Work out the finished part from the listing and answer in its coordinate system (mm). A direction names the side the tool comes from. Round coordinates to 2 decimals unless told otherwise and drop trailing zeros. Write each loop counter-clockwise with the first axis right and the second up, starting at its lowest first coordinate (ties: lowest second). Pieces come first, ordered by that corner, then holes. Notation, with made-up numbers: M -15.5,-25 L 1.5,-25 A27 ccw 1.5,-7 Z; hole C -20.75,-26 d5. An arc over 180 degrees is marked long. One line per item, written item: value. Start each with the question number.
Q1. Find section A-A (x = 99.5). Write down the section's boundary in (y, z), and give its area (3 significant figures).
Q2. A tool of negligible diameter and unlimited length cuts with its end or side. For faces 4 (the flat face through (-5.5, 6, -65)), 5 (the flat face through (16, 6, 45.156)), 6 (the flat face through (57, 6, 45.156)), from which of +Z, -Z, +X, -X, +Y, -Y can it reach the whole face along a straight path? Write none if from no direction.
Q3. Consider probe 1 along X at (y, z) = (1.75, -117); probe 2 along X at (y, z) = (6, -40); probe 3 along Y at (x, z) = (11, 39). Determine where each line is inside the solid, lowest interval first.
Q4. Find section B-B (z = -69). Write down the section's boundary in (x, y), and give its area (3 significant figures).
Q5. Given pin 1 Ø3 at (x, y) = (12.5, 7) entering from +Z; pin 2 Ø1.8 at (y, z) = (6, 28.41) entering from +X; pin 3 Ø1.5 at (y, z) = (1.5, -28) entering from -X, each flat-ended and moving along its own axis, determine where each tip first touches the part or whether it passes through.
Q6. The mould has two halves that part along X. Classify faces 1 (the flat face through (73.5, 6, 40)), 2 (the flat face through (28, 6, 52)), 3 (the flat face through (-12, 6, -0.344)): released by +X, released by -X, zero draft, split by the parting line, or undercut.
from build123d import *

# Parameters (mm, degrees)
BOSS_EXTRUDE1_DEPTH = 12
SKETCH2_R           = 0.9921875
CUT_EXTRUDE1_DEPTH  = 12
SKETCH3_R           = 0.9921875
CUT_EXTRUDE2_DEPTH  = 12
SKETCH4_R           = 1
CUT_EXTRUDE3_DEPTH  = 219.054378342


with BuildPart() as part:
    # Sketch1 → Boss-Extrude1 (new body)
    with BuildSketch(Plane(origin=(0, 0, 0), x_dir=(1, 0, 0), z_dir=(0, 1, 0))):
        with BuildLine():
            Line((-5.5, 132.84375), (-5.5, 94.34375))
            Line((-5.5, 94.34375), (-17.5, 94.34375))
            Line((-17.5, 94.34375), (-17.5, 82.34375))
            Line((-17.5, 82.34375), (-5.5, 82.34375))
            Line((-5.5, 82.34375), (-5.5, 48.84375))
            Line((-5.5, 48.84375), (4.5, 48.84375))
            Line((4.5, 48.84375), (4.5, 33.84375))
            Line((4.5, 33.84375), (-5.5, 33.84375))
            Line((-5.5, 33.84375), (-5.5, 0.34375))
            Line((-5.5, 0.34375), (-17.5, 0.34375))
            Line((-17.5, 0.34375), (-17.5, -11.65625))
            Line((-17.5, -11.65625), (-5.5, -11.65625))
            Line((-5.5, -11.65625), (-5.5, -35.15625))
            ThreePointArc((-5.5, -35.15625), (-2.571067812, -42.227317812), (4.5, -45.15625))
            Line((4.5, -45.15625), (28, -45.15625))
            Line((28, -45.15625), (28, -57.15625))
            Line((28, -57.15625), (40, -57.15625))
            Line((40, -57.15625), (40, -45.15625))
            Line((40, -45.15625), (73.5, -45.15625))
            Line((73.5, -45.15625), (73.5, -35.15625))
            Line((73.5, -35.15625), (88.5, -35.15625))
            Line((88.5, -35.15625), (88.5, -45.15625))
            Line((88.5, -45.15625), (122, -45.15625))
            Line((122, -45.15625), (122, -57.15625))
            Line((122, -57.15625), (134, -57.15625))
            Line((134, -57.15625), (134, -45.15625))
            Line((134, -45.15625), (172.5, -45.15625))
            Line((172.5, -45.15625), (172.5, -31.15625))
            ThreePointArc((172.5, -31.15625), (169.571067812, -24.085182188), (162.5, -21.15625))
            Line((162.5, -21.15625), (68.5, -21.15625))
            ThreePointArc((68.5, -21.15625), (33.144660941, -6.511589059), (18.5, 28.84375))
            Line((18.5, 28.84375), (18.5, 122.84375))
            ThreePointArc((18.5, 122.84375), (15.571067812, 129.914817812), (8.5, 132.84375))
            Line((8.5, 132.84375), (-5.5, 132.84375))
        make_face()
    extrude(amount=BOSS_EXTRUDE1_DEPTH)

    # Sketch2 → Cut-Extrude1 (cut)
    with BuildSketch(Plane.XY.offset(45.15625)):
        with Locations((153.25, 6)):
            Circle(SKETCH2_R)
        with Locations((11.25, 6)):
            Circle(SKETCH2_R)
    extrude(amount=-CUT_EXTRUDE1_DEPTH, mode=Mode.SUBTRACT)

    # Sketch3 → Cut-Extrude2 (cut)
    with BuildSketch(Plane.ZY.offset(5.5)):
        with Locations((28.40625, 6)):
            Circle(SKETCH3_R)
        with Locations((-113.59375, 6)):
            Circle(SKETCH3_R)
    extrude(amount=-CUT_EXTRUDE2_DEPTH, mode=Mode.SUBTRACT)

    # Sketch4 → Cut-Extrude3 (cut, through all)
    with BuildSketch(Plane(origin=(0, 0, 0), x_dir=(1, 0, 0), z_dir=(0, 1, 0))):
        with Locations((-5.5, 94.34375)):
            Circle(SKETCH4_R)
        with Locations((-5.5, 82.34375)):
            Circle(SKETCH4_R)
        with Locations((-5.5, 0.34375)):
            Circle(SKETCH4_R)
        with Locations((-5.5, -11.65625)):
            Circle(SKETCH4_R)
        with Locations((28, -45.15625)):
            Circle(SKETCH4_R)
        with Locations((40, -45.15625)):
            Circle(SKETCH4_R)
        with Locations((122, -45.15625)):
            Circle(SKETCH4_R)
        with Locations((134, -45.15625)):
            Circle(SKETCH4_R)
    extrude(amount=CUT_EXTRUDE3_DEPTH, mode=Mode.SUBTRACT)


solid = part.part
The answers:
1. outline: M 0,21.16 L 12,21.16 L 12,45.16 L 0,45.16 Z
1. area: 288 mm2
2. face 4: -X, +Y, -Y
2. face 5: +Z, -X, +Y, -Y
2. face 6: +Z, +Y, -Y
3. probe 1: -5.5 to 18.5
3. probe 2: 4.5 to 18.5
3. probe 3: 0 to 5.04, 6.96 to 12
4. outline: M -5.5,0 L 18.5,0 L 18.5,12 L -5.5,12 Z
4. area: 288 mm2
5. pin 1: z = 45.16
5. pin 2: x = 172.33
5. pin 3: x = -5.5
6. face 1: undercut
6. face 2: released by -X
6. face 3: zero draft
